Source: CAD feature listing. Evaluate the final solid. Frame: model axes, mm. A direction names the side the tool comes from. Give positions to 0.01 mm unless a question says otherwise; leave off trailing zeros. Write each loop counter-clockwise with the first axis right and the second up, starting at its lowest first coordinate (ties: lowest second). Pieces come first, ordered by that corner, then holes. Notation, with made-up numbers: (10, 60.5) - (40, 60.5) arc R13 cw to (40, 75.5) - close; hole circle Ø6 at (-1.5, -5.5). An arc over 180 degrees is marked (long way). Answer as a JSON object with one key per item and string values. Group by question number.
from build123d import *

# Parameters (mm, degrees)
SKETCH1_R           = 8.5
SKETCH1_R_2         = 4
BOSS_EXTRUDE1_DEPTH = 8


with BuildPart() as part:
    # Sketch1 → Boss-Extrude1 (new body)
    with BuildSketch(Plane.XY):
        with BuildLine():
            ThreePointArc((7.5, -14.696938457), (0, 16.5), (-7.5, -14.696938457))
            Line((-7.5, -14.696938457), (-7.5, -30.078432584))
            ThreePointArc((-7.5, -30.078432584), (-3.75, -40), (-7.5, -49.921567416))
            Line((-7.5, -49.921567416), (-7.5, -147.482509157))
            Line((-7.5, -147.482509157), (0, -147.482509157))
            ThreePointArc((0, -147.482509157), (36.911874913, -178.286162824), (13.210921757, -220.114579102))
            ThreePointArc((13.210921757, -220.114579102), (-16.280138823, -232.684600513), (15.685388352, -235.120409383))
            ThreePointArc((15.685388352, -235.120409383), (52.349526518, -180.803106174), (7.5, -133.020803734))
            Line((7.5, -133.020803734), (7.5, -49.921567416))
            ThreePointArc((7.5, -49.921567416), (3.75, -40), (7.5, -30.078432584))
            Line((7.5, -30.078432584), (7.5, -14.696938457))
        make_face()
        with Locations((0, -230)):
            Circle(SKETCH1_R, mode=Mode.SUBTRACT)
        with Locations((0, -65)):
            Circle(SKETCH1_R_2, mode=Mode.SUBTRACT)
        Circle(SKETCH1_R, mode=Mode.SUBTRACT)
    extrude(amount=BOSS_EXTRUDE1_DEPTH)


solid = part.part
Q1. First-contact query: pin 1 Ø2 at (x, z) = (3, 1.5) entering from -Y; pin 2 Ø1.5 at (y, z) = (-208.5, 7) entering from -X; pin 3 Ø2 at (y, z) = (-203, 3) entering from +X. Flat tips, straight axial feed; report the tip coordinate or a pass-through.
Q2. Reachability of faces 1 (the flat face through (-7.5, -22, 4)), 2 (the flat face through (7.5, -22, 4)), 3 (the cylindrical face through (-1.107, -221.572, 3.944)) from +Z, -Z, +X, -X, +Y, -Y: full face, straight path, thin tool, end or side. Return the list, or none.
Q3. Section A-A on y = 0. Return the cut outline in (x, z), then the cut area to 3 significant figures.
Q4. Draft query along Y for faces 4 (the cylindrical face through (36.774, -177.569, 3.944)), 5 (the flat face through (-7.5, -98, 4)), 6 (the flat face through (10, -134, 8)). Return one class per face: released by +Y, released by -Y, zero draft, split by the parting line, or undercut.
Q5. Section B-B on z = 4. Return the cut outline in (x, y).
Q6. Section D-D on x = 40. Return the cut outline in (y, z).
Q7. Section C-C on y = -230. Return the cut outline in (x, z), then the cut area to 3 significant figures.
Q8. Ray query, probe 1 along Y at (x, z) = (11, 4); probe 2 along Y at (x, z) = (-5.5, 6.25); probe 3 along Y at (x, z) = (0.5, 5). Return the intervals inside material, ascending. Write a range as [from, to].
Taken from the geometry:
{
 "1": {"pin 1": "stops at y = -246.38", "pin 2": "stops at x = 28.63", "pin 3": "stops at x = 49.69"},
 "2": {"face 1": "+Z, -Z, -X", "face 2": "+Z, -Z, +X", "face 3": "+Z, -Z"},
 "3": {"outline": "(-16.5, 0) - (-8.5, 0) - (-8.5, 8) - (-16.5, 8) - close; (8.5, 0) - (16.5, 0) - (16.5, 8) - (8.5, 8) - close", "area": "128 mm²"},
 "4": {"face 4": "undercut", "face 5": "undercut", "face 6": "zero draft"},
 "5": {"outline": "(-7.5, -147.48) - (0, -147.48) arc R37.52 cw to (13.21, -220.11) arc R16.5 ccw (long way) to (15.69, -235.12) arc R52.52 ccw to (7.5, -133.02) - (7.5, -49.92) arc R15 cw to (7.5, -30.08) - (7.5, -14.7) arc R16.5 ccw (long way) to (-7.5, -14.7) - (-7.5, -30.08) arc R15 cw to (-7.5, -49.92) - close; hole circle Ø17 at (0, -230); hole circle Ø17 at (0, 0); hole circle Ø8 at (0, -65)"},
 "6": {"outline": "(-219.03, 0) - (-150.97, 0) - (-150.97, 8) - (-219.03, 8) - close"},
 "7": {"outline": "(-16.5, 0) - (-8.5, 0) - (-8.5, 8) - (-16.5, 8) - close; (8.5, 0) - (27.08, 0) - (27.08, 8) - (8.5, 8) - close", "area": "213 mm²"},
 "8": {"probe 1": "y = [-242.3, -217.7], [-149.13, -133.65], [-12.3, 12.3]", "probe 2": "y = [-245.56, -236.48], [-223.52, -214.44], [-147.48, -47.03], [-32.97, -6.48], [6.48, 15.56]", "probe 3": "y = [-246.49, -238.49], [-221.51, -213.51], [-147.49, -68.97], [-61.03, -8.49], [8.49, 16.49]"}
}
